Could you check a few things on this model? Use its own coordinates, in mm. A direction names the side the tool comes from. Give positions to 0.01 mm unless a question says otherwise; leave off trailing zeros. Write each loop counter-clockwise with the first axis right and the second up, starting at its lowest first coordinate (ties: lowest second). Pieces come first, ordered by that corner, then holes. Notation, with made-up numbers: M 56.5,47 L 97.5,47 A20 cw 97.5,61 Z; hole C 30,64.5 d7. An arc over 180 degrees is marked long. Answer as CSV lines item,"result". Start each with the question number.
from build123d import *

# Parameters (mm, degrees)
SKETCH1_R           = 15
BOSS_EXTRUDE1_DEPTH = 20
BOSS_EXTRUDE2_DEPTH = 20
CIRPATTERN1_COUNT   = 18
SKETCH3_R           = 1
BOSS_EXTRUDE3_DEPTH = 2
SKETCH4_R           = 1
BOSS_EXTRUDE4_DEPTH = 2


with BuildPart() as part:
    # Sketch1 → Boss-Extrude1 (new body)
    with BuildSketch(Plane.XY):
        Circle(SKETCH1_R)
    extrude(amount=BOSS_EXTRUDE1_DEPTH)

    # Sketch2 → Boss-Extrude2 (add)
    with BuildSketch(Plane.XY.offset(20)):
        Polygon((0, 17), (1, 17), (2, 13), (0, 13), (-2, 13), (-1, 17), align=None)
    boss_extrude2 = extrude(amount=-BOSS_EXTRUDE2_DEPTH)

    # CirPattern1: Boss-Extrude2 ×18 about axis
    cirpattern1_axis = Axis((0, 0, 0), (0, 0, 1))
    for i in range(1, CIRPATTERN1_COUNT):
        add(boss_extrude2.rotate(cirpattern1_axis, i * 360 / CIRPATTERN1_COUNT))

    # Sketch3 → Boss-Extrude3 (add)
    with BuildSketch(Plane(origin=(0, 0, 0), x_dir=(-1, 0, 0), z_dir=(0, 0, -1))):
        Circle(SKETCH3_R)
    extrude(amount=BOSS_EXTRUDE3_DEPTH)

    # Sketch4 → Boss-Extrude4 (add)
    with BuildSketch(Plane.XY.offset(20)):
        Circle(SKETCH4_R)
    extrude(amount=BOSS_EXTRUDE4_DEPTH)


solid = part.part
1. Will these pins go through, and if not, where does the flat tip stop? P1, Ø8, axis at y = -6, z = 4, coming from the -X side; P2, Ø10, axis at x = -8.5, y = 7, coming from the -Z side; P3, Ø4, axis at y = -6.5, z = 18, coming from the +X side.
2. Imagine slicing it at C-C, the plane y = 13. Please give me the cut outline in (x, z).
3. Imagine slicing it at A-A, the plane y = 0. Please give me the cut outline in (x, z), plus the area to 3 significant figures.
4. On a 3-axis mill with a long thin cutter (end or side, diameter ignored), from which of +Z, -Z, +X, -X, +Y, -Y can I reach the whole of each face in a straight line? I mean faces 5 (the flat face through (1.263, -15.947, 10.14)), 6 (the flat face through (16.74, -2.97, 10.14)), 7 (the cylindrical face through (-2.59, 14.775, 9.86)), 8 (the flat face through (-14.464, -6.9, 10.14)). Say none if no direction works.
5. Imagine slicing it at D-D, the plane y = -11.5. Please give me the cut outline in (x, z).
6. Thinking about a two-plate mould opening in Y: for faces 1 (the cylindrical face through (0, -1, 21)), 2 (the flat face through (-5.83, -15.97, 10.14)), 3 (the cylindrical face through (15, 0, 10)), 4 (the flat face through (-14.715, 8.512, 10.14)), which applies, pulls with the +Y half, pulls with the -Y half, needs draft (parallel to the pull), parting line crosses it, or undercut?
7. Please list where these lines run through material, in increasing order: line 1 (X direction, y = -15, z = 11.25); line 2 (Y direction, x = -11.5, z = 9.5); line 3 (Z direction, x = -7.5, y = 9.5).
8. Imagine slicing it at B-B, the plane x = 0. Please give me the cut outline in (y, z).
Solutions:
1,P1,"x = -16.91"
1,P2,"z = 0"
1,P3,"x = 15.22"
2,outline,"M -10.95,0 L -9.24,0 L -9.24,20 L -10.95,20 Z; M -7.48,0 L 7.48,0 L 7.48,20 L -7.48,20 Z; M 9.24,0 L 10.95,0 L 10.95,20 L 9.24,20 Z"
3,outline,"M -15,0 L -1,0 L -1,-2 L 1,-2 L 1,0 L 15,0 L 15,20 L 1,20 L 1,22 L -1,22 L -1,20 L -15,20 Z"
3,area,"608 mm²"
4,face 5,"+Z, -Z, -Y"
4,face 6,"+Z, -Z, +X, -Y"
4,face 7,"+Z, -Z, +Y"
4,face 8,"+Z, -Z, -X"
5,outline,"M -11.26,0 L 11.26,0 L 11.26,20 L -11.26,20 Z"
6,face 1,"parting line crosses it"
6,face 2,"pulls with the -Y half"
6,face 3,"undercut"
6,face 4,"pulls with the +Y half"
7,line 1,"-6.69 to -3.99, -1.5 to 1.5, 3.99 to 6.69"
7,line 2,"-12.54 to -11.98, -9.63 to 9.63, 11.98 to 12.54"
7,line 3,"0 to 20"
8,outline,"M -17,0 L -1,0 L -1,-2 L 1,-2 L 1,0 L 17,0 L 17,20 L 1,20 L 1,22 L -1,22 L -1,20 L -17,20 Z"
